The drawing under review shows one solid part. Ordinate dimensions are in mm from its lowest x, y, z. Coordinates: 2 decimals unless noted, no trailing zeros. Order: outer loops, then holes, each group sorted by start corner. A loop starts at its lowest first (then second) coordinate and runs counter-clockwise, first axis right, second up. Notation, with made-up numbers: (9, -6.5) -> (28, -6.5) arc R13 cw to (28, 12.5) -> close; hole circle Ø1 at (-11.5, 64.25). An arc over 180 degrees is marked (long way). Put each result on its own line as item: value.
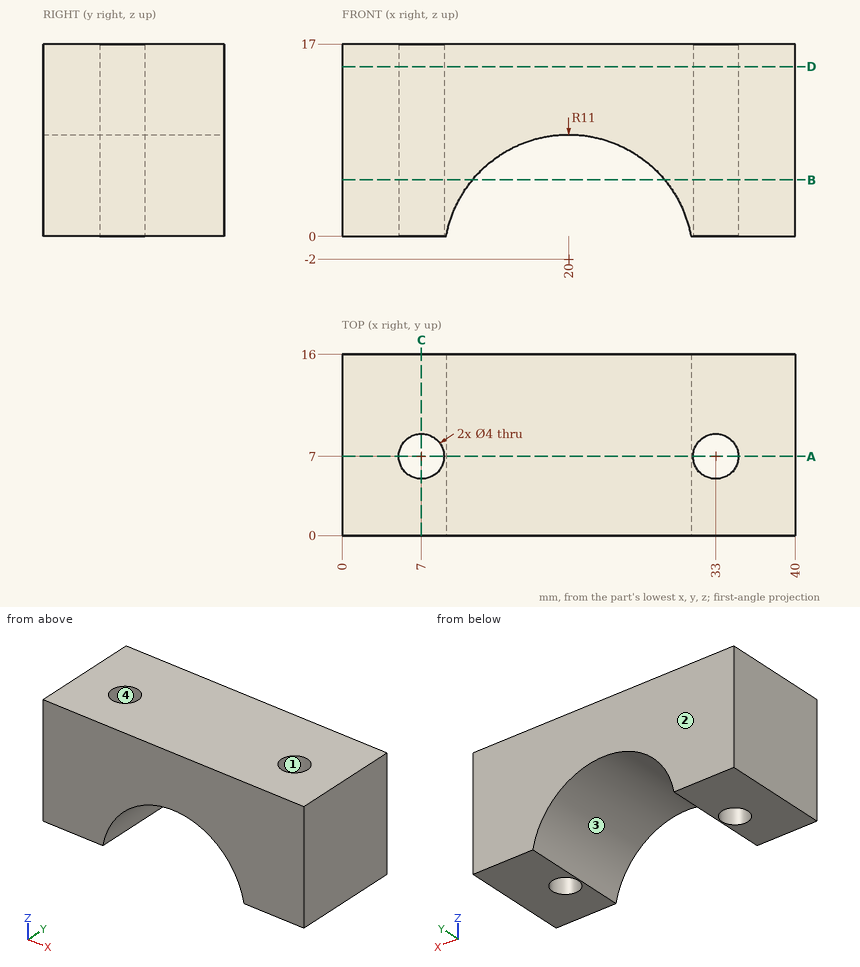
Item 1: Mouldability with a two-part tool opening along Y and no side actions: class the marked faces 1, 2, 3 and 4 as +Y half, -Y half, draft (parallel to the pull), parting line (faces both ways), or undercut.
Answers below:
face 1: undercut
face 2: +Y half
face 3: draft
face 4: undercut
Item 2: Consider section A-A on y = 7. Write out the cut boundary in (x, z), and give its area (3 significant figures).
Answers below:
outline: (0, 0) -> (5, 0) -> (5, 17) -> (0, 17) -> close; (9, 0) -> (9.18, 0) arc R11 cw to (30.82, 0) -> (31, 0) -> (31, 17) -> (9, 17) -> close; (35, 0) -> (40, 0) -> (40, 17) -> (35, 17) -> close
area: 398 mm^2
Item 3: For line 1 (Y direction, x = 33, z = 10); line 2 (X direction, y = 2.75, z = 4); line 3 (Z direction, x = 24, y = 5.5), list the stretches that pass through material, from the lowest coordinate up. Write a range as from..to.
Answers below:
line 1: 0..5, 9..16
line 2: 0..10.78, 29.22..40
line 3: 8.25..17
Item 4: Consider section B-B on z = 5. Write out the cut boundary in (x, y), and give its area (3 significant figures).
Answers below:
outline: (0, 0) -> (11.51, 0) -> (11.51, 16) -> (0, 16) -> close; (28.49, 0) -> (40, 0) -> (40, 16) -> (28.49, 16) -> close; hole circle Ø4 at (7, 7); hole circle Ø4 at (33, 7)
area: 343 mm^2
Item 5: Consider section C-C on x = 7. Write out the cut boundary in (y, z).
Answers below:
outline: (0, 0) -> (5, 0) -> (5, 17) -> (0, 17) -> close; (9, 0) -> (16, 0) -> (16, 17) -> (9, 17) -> close
Item 6: For pin 1 Ø5 at (x, y) = (33, 7) entering from -Z, flat-tipped, find the tip position at first contact; note if it passes through.
Answers below:
pin 1: z = 0
Item 7: Consider section D-D on z = 15. Write out the cut boundary in (x, y).
Answers below:
outline: (0, 0) -> (40, 0) -> (40, 16) -> (0, 16) -> close; hole circle Ø4 at (7, 7); hole circle Ø4 at (33, 7)
